from build123d import *

# Parameters (mm, degrees)
SKETCH4_R           = 4.826
SKETCH4_R_2         = 7.62
BOSS_EXTRUDE3_DEPTH = 152.4
SKETCH5_W           = 22.225
SKETCH5_H           = 22.225
SKETCH5_W_2         = 25.4
SKETCH5_H_2         = 101.6
CUT_EXTRUDE2_DEPTH  = 258.622422
SKETCH6_W           = 25.4
SKETCH6_H           = 101.6
SKETCH6_W_2         = 22.225
SKETCH6_H_2         = 22.225
CUT_EXTRUDE3_DEPTH  = 123.590867
CUT_EXTRUDE4_DEPTH  = 152.4
SKETCH8_R           = 6.35
BOSS_EXTRUDE4_DEPTH = 101.6
SKETCH9_W           = 25.4
SKETCH9_H           = 25.4
SKETCH9_W_2         = 22.225
SKETCH9_H_2         = 22.225
BOSS_EXTRUDE5_DEPTH = 58.928
SKETCH11_R          = 1.65
CUT_EXTRUDE6_DEPTH  = 1.5875
SKETCH12_R          = 6.35
CUT_EXTRUDE7_DEPTH  = 103.1875
SKETCH13_W          = 25.4
SKETCH13_H          = 25.4
SKETCH13_W_2        = 22.225
SKETCH13_H_2        = 22.225
BOSS_EXTRUDE6_DEPTH = 68.072
SKETCH14_R          = 3.33
SKETCH14_R_2        = 3.42
CUT_EXTRUDE8_DEPTH  = 1.5875


with BuildPart() as part:
    # Sketch4 → Boss-Extrude3 (new body)
    with BuildSketch(Plane(origin=(0, 0, 0), x_dir=(1, 0, 0), z_dir=(0, 1, 0))):
        Polygon((-254, -12.7), (-254, 12.7), (-4.622421975, 12.7), (82.971713376, 86.200206667), (99.298518662, 66.742677811), (4.622421975, -12.7), align=None)
        Circle(SKETCH4_R, mode=Mode.SUBTRACT)
        with Locations((63.236968779, 53.06211718)):
            Circle(SKETCH4_R, mode=Mode.SUBTRACT)
        with Locations((-228.6, 0)):
            Circle(SKETCH4_R_2, mode=Mode.SUBTRACT)
    extrude(amount=BOSS_EXTRUDE3_DEPTH)

    # Sketch5 → Cut-Extrude2 (cut)
    with BuildSketch(Plane.ZY.offset(254)):
        with Locations((0, 139.7)):
            Rectangle(SKETCH5_W, SKETCH5_H)
        with Locations((0, 76.2)):
            Rectangle(SKETCH5_W_2, SKETCH5_H_2)
        with Locations((0, 12.7)):
            Rectangle(SKETCH5_W, SKETCH5_H)
    extrude(amount=-CUT_EXTRUDE2_DEPTH, mode=Mode.SUBTRACT)

    # Sketch6 → Cut-Extrude3 (cut)
    with BuildSketch(Plane(origin=(91.135116019, 0, -76.471442239), x_dir=(-0.64278761, 0, -0.766044443), z_dir=(0.766044443, 0, -0.64278761))):
        with Locations((0, 76.2)):
            Rectangle(SKETCH6_W, SKETCH6_H)
        with Locations((0, 139.7)):
            Rectangle(SKETCH6_W_2, SKETCH6_H_2)
        with Locations((0, 12.7)):
            Rectangle(SKETCH6_W_2, SKETCH6_H_2)
    extrude(amount=-CUT_EXTRUDE3_DEPTH, mode=Mode.SUBTRACT)

    # Sketch7 → Cut-Extrude4 (cut)
    with BuildSketch(Plane(origin=(0, 152.4, 0), x_dir=(1, 0, 0), z_dir=(0, 1, 0))):
        with BuildLine():
            Line((55.073566136, 62.790881607), (14.292485888, 190.379547218))
            Line((14.292485888, 190.379547218), (153.844328146, 116.591677596))
            Line((153.844328146, 116.591677596), (141.535463421, -3.473116834))
            Line((141.535463421, -3.473116834), (71.400371422, 43.333352752))
            ThreePointArc((71.400371422, 43.333352752), (72.965733207, 61.225519823), (55.073566136, 62.790881607))
        make_face()
    extrude(amount=-CUT_EXTRUDE4_DEPTH, mode=Mode.SUBTRACT)

    # Sketch8 → Boss-Extrude4 (add)
    with BuildSketch(Plane.XZ.offset(-127)):
        with Locations((-76.2, 0)):
            Circle(SKETCH8_R)
        with Locations((-152.4, 0)):
            Circle(SKETCH8_R)
    extrude(amount=BOSS_EXTRUDE4_DEPTH)

    # Sketch9 → Boss-Extrude5 (add)
    with BuildSketch(Plane.ZY.offset(254)):
        with Locations((0, 139.7)):
            Rectangle(SKETCH9_W, SKETCH9_H)
        with Locations((0, 139.7)):
            Rectangle(SKETCH9_W_2, SKETCH9_H_2, mode=Mode.SUBTRACT)
        with Locations((0, 12.7)):
            Rectangle(SKETCH9_W, SKETCH9_H)
        with Locations((0, 12.7)):
            Rectangle(SKETCH9_W_2, SKETCH9_H_2, mode=Mode.SUBTRACT)
    extrude(amount=BOSS_EXTRUDE5_DEPTH)

    # Sketch11 → Cut-Extrude6 (cut)
    with BuildSketch(Plane.XZ.offset(-127)):
        with Locations((-271.054789466, 0)):
            Circle(SKETCH11_R)
        with Locations((-296.054789466, 0)):
            Circle(SKETCH11_R)
    extrude(amount=-CUT_EXTRUDE6_DEPTH, mode=Mode.SUBTRACT)

    # Sketch12 → Cut-Extrude7 (cut)
    with BuildSketch(Plane.XZ.offset(-127)):
        with Locations((-283.554789466, 0)):
            Circle(SKETCH12_R)
    extrude(amount=CUT_EXTRUDE7_DEPTH, mode=Mode.SUBTRACT)

    # Sketch13 → Boss-Extrude6 (add)
    with BuildSketch(Plane.ZY.offset(312.928)):
        with Locations((0, 139.7)):
            Rectangle(SKETCH13_W, SKETCH13_H)
        with Locations((0, 139.7)):
            Rectangle(SKETCH13_W_2, SKETCH13_H_2, mode=Mode.SUBTRACT)
    extrude(amount=BOSS_EXTRUDE6_DEPTH)

    # Sketch14 → Cut-Extrude8 (cut)
    with BuildSketch(Plane.XY.offset(12.7)):
        with Locations((-370.26, 136.87)):
            Circle(SKETCH14_R)
        with Locations((-283.26, 136.87)):
            Circle(SKETCH14_R)
        with Locations((-301.58, 19.63)):
            Circle(SKETCH14_R_2)
    extrude(amount=-CUT_EXTRUDE8_DEPTH, mode=Mode.SUBTRACT)


solid = part.part
The listing builds one solid part. Answer for the finished solid, in the listing's coordinates (mm). A direction names the side the tool comes from. Coordinates: 2 decimals unless noted, no trailing zeros. Write each loop counter-clockwise with the first axis right and the second up, starting at its lowest first coordinate (ties: lowest second). Pieces come first, ordered by that corner, then holes. Notation, with made-up numbers: (-17.5, -33) -> (-8.5, -33) arc R31 ccw to (-8.5, -4) -> close; hole circle Ø4 at (-35, 78.25). An arc over 180 degrees is marked (long way). One line per question, with ' | ' between items.
1. Section C-C (x = -228.6) is taken. State how many separate pieces and enclosed holes the cut face has, and give its area (3 significant figures).
Verdict:
separate pieces: 4 | enclosed holes: 0 | area: 206 mm^2
2. Section D-D (x = -152.4) is taken. Determine the outline of the cut face in (y, z), and give its area (3 significant figures).
Verdict:
outline: (0, -12.7) -> (25.4, -12.7) -> (25.4, -6.35) -> (127, -6.35) -> (127, -12.7) -> (152.4, -12.7) -> (152.4, 12.7) -> (127, 12.7) -> (127, 6.35) -> (25.4, 6.35) -> (25.4, 12.7) -> (0, 12.7) -> close; hole (1.59, -11.11) -> (23.81, -11.11) -> (23.81, 11.11) -> (1.59, 11.11) -> close; hole (128.59, -11.11) -> (150.81, -11.11) -> (150.81, 11.11) -> (128.59, 11.11) -> close | area: 1,590 mm^2
3. For a pull along Y with two mould halves and no side action, classify faces 4 (the flat face through (-151, 152.4, -6)), 5 (the cylindrical face through (67.84, 24.6, -54.51)), 6 (the flat face through (-190, 140, -11.112)) as released by +Y, released by -Y, zero draft, split by the parting line, or undercut.
Verdict:
face 4: released by +Y | face 5: zero draft | face 6: undercut
4. Section B-B (y = 9.5) is taken. Determine the outline of the cut face in (x, z), and give its area (3 significant figures).
Verdict:
outline: (-312.93, -12.7) -> (-4.62, -12.7) -> (55.07, -62.79) arc R12.7 ccw to (60.8, -65.53) -> (-4.04, -11.11) -> (-312.93, -11.11) -> close; (-312.93, 11.11) -> (3.29, 11.11) -> (3.6, 11.48) -> (4.04, 11.11) -> (4.62, 11.11) -> (4.62, 10.63) -> (75.09, -48.5) arc R12.7 ccw to (71.4, -43.33) -> (4.62, 12.7) -> (-312.93, 12.7) -> close | area: 1,270 mm^2
5. Given pin 1 Ø12 at (y, z) = (75, -5.5) entering from +X; pin 2 Ø15.5 at (x, z) = (63.24, -53.06) entering from -Y; pin 3 Ø6 at (y, z) = (136.5, -25) entering from -X; pin 4 Ø12 at (x, z) = (-228.6, 0) entering from -Y, each flat-ended and moving along its own axis, determine where each tip first touches the part or whether it passes through.
Verdict:
pin 1: stops at x = -69.85 | pin 2: stops at y = 0 | pin 3: stops at x = 6.46 | pin 4: passes through
6. Section A-A (x = -48.5) is taken. Determine the outline of the cut face in (y, z), and give its area (3 significant figures).
Verdict:
outline: (0, -12.7) -> (25.4, -12.7) -> (25.4, 12.7) -> (0, 12.7) -> close; (127, -12.7) -> (152.4, -12.7) -> (152.4, 12.7) -> (127, 12.7) -> close; hole (1.59, -11.11) -> (23.81, -11.11) -> (23.81, 11.11) -> (1.59, 11.11) -> close; hole (128.59, -11.11) -> (150.81, -11.11) -> (150.81, 11.11) -> (128.59, 11.11) -> close | area: 302 mm^2
7. Which of the six approach directions +Z, -Z, +X, -X, +Y, -Y give full straight-line access (tool end or side, diameter ignored) to faces 1 (the flat face through (-161, 13, -12.7)), 2 (the flat face through (-153, 13, 11.112)), 3 (the flat face through (40.35, 139.54, -19.35))?
Verdict:
face 1: -Z, -X, +Y, -Y | face 2: -X | face 3: none
8. Straight lines are drawn through the part: line 1 (Y direction, x = -46.5, z = 6); line 2 (Z direction, x = -228, y = 1); line 3 (X direction, y = 151, z = 0). For each, find the intervals that lie inside material, in ascending order.
Verdict:
line 1: y = 0 to 1.59, 23.81 to 25.4, 127 to 128.59, 150.81 to 152.4 | line 2: z = -12.7 to -7.6, 7.6 to 12.7 | line 3: x = -381 to -236.22, -220.98 to -4.83, 4.83 to 19.76
